```python
from build123d import *

# Parameters (mm, degrees)
EXTRUDE_1_DEPTH     = 20
SKETCH_2_W          = 23.1
SKETCH_2_H          = 23.1
SKETCH_2_W_2        = 15.1
SKETCH_2_H_2        = 15.1
EXTRUDE_2_DEPTH     = 24
SKETCH_3_W          = 4
SKETCH_3_H          = 23.1
EXTRUDE_3_DEPTH     = 15
SKETCH_4_R          = 1.8
CUT_EXTRUDE_1_DEPTH = 15
SKETCH_5_R          = 1.8
CUT_EXTRUDE_2_DEPTH = 35
SKETCH_6_W          = 23.1
SKETCH_6_H          = 19
CUT_EXTRUDE_3_DEPTH = 2


with BuildPart() as part:
    # 草图1 → 凸台-拉伸1 (new body)
    with BuildSketch(Plane(origin=(0, 0, 0), x_dir=(1, 0, 0), z_dir=(0, 1, 0))):
        Polygon((-11.153846154, 14.269230769), (-7.153846154, 14.269230769), (-7.153846154, -0.730769231), (7.946153846, -0.730769231), (7.946153846, 14.269230769), (11.946153846, 14.269230769), (11.946153846, -0.730769231), (11.946153846, -4.730769231), (-7.384615385, -4.730769231), (-11.153846154, -4.730769231), align=None)
    extrude(amount=EXTRUDE_1_DEPTH)

    # 草图2 → 凸台-拉伸2 (add)
    with BuildSketch(Plane(origin=(0, 0, 0.730769231), x_dir=(-1, 0, 0), z_dir=(0, 0, -1))):
        with Locations((-0.396153846, -11.55)):
            Rectangle(SKETCH_2_W, SKETCH_2_H)
        with Locations((-0.396153846, -11.55)):
            Rectangle(SKETCH_2_W_2, SKETCH_2_H_2, mode=Mode.SUBTRACT)
    extrude(amount=-EXTRUDE_2_DEPTH)

    # 草图3 → 凸台-拉伸3 (add)
    with BuildSketch(Plane(origin=(0, 0, 0.730769231), x_dir=(-1, 0, 0), z_dir=(0, 0, -1))):
        with Locations((-9.946153846, -11.55)):
            Rectangle(SKETCH_3_W, SKETCH_3_H)
        with Locations((9.153846154, -11.55)):
            Rectangle(SKETCH_3_W, SKETCH_3_H)
    extrude(amount=EXTRUDE_3_DEPTH)

    # 草图4 → 切除-拉伸1 (cut)
    with BuildSketch(Plane.XY.offset(4.730769231)):
        with Locations((0, 12.5)):
            Circle(SKETCH_4_R)
    extrude(amount=-CUT_EXTRUDE_1_DEPTH, mode=Mode.SUBTRACT)

    # 草图5 → 切除-拉伸2 (cut)
    with BuildSketch(Plane(origin=(11.946153846, 0, 0), x_dir=(0, 0, -1), z_dir=(1, 0, 0))):
        with Locations((-17.230769231, -11.5)):
            Circle(SKETCH_5_R)
    extrude(amount=-CUT_EXTRUDE_2_DEPTH, mode=Mode.SUBTRACT)

    # 草图6 → 切除-拉伸3 (cut)
    with BuildSketch(Plane(origin=(0, 20, 0), x_dir=(1, 0, 0), z_dir=(0, 1, 0))):
        with Locations((0.396153846, 4.769230769)):
            Rectangle(SKETCH_6_W, SKETCH_6_H)
    extrude(amount=-CUT_EXTRUDE_3_DEPTH, mode=Mode.SUBTRACT)


solid = part.part
```
For this review, take the finished solid that the model builds, in its own axes (mm). A direction names the side the tool comes from. Give positions to 0.01 mm unless a question says otherwise; leave off trailing zeros. Loops run counter-clockwise (first coordinate to the right, second up) from the corner with the lowest first, then second, coordinate; pieces in that order, holes last. Notation, with made-up numbers: M 19.25,-12 L 63.25,-12 A19 ccw 63.25,0 Z; hole C 10.5,89 d4. An arc over 180 degrees is marked long. One line per item, written item: value. Start each with the question number.
Q1. Add section D-D (y = 12.5). Give the boundary of the cut face in (x, z), and give its area (3 significant figures).
Q2. Add section B-B (x = 2.75). Give the boundary of the cut face in (y, z), and give its area (3 significant figures).
Q3. Add section A-A (y = -11.5). Give the boundary of the cut face in (x, z).
Q4. For L1, parallel to Y at x = 0, z = 3.75; L2, parallel to X at y = -16, z = 16.5; L3, parallel to Y at x = -5, z = 16, list the stretches that pass through material, from the lowest coordinate up.
Q5. Draft analysis for pull direction Y (two halves, no side actions). For faces 1 (the face through (-9.13, -11.42, 19.03)), 2 (the face through (1, 0, 15)), 3 (the face through (-7.154, -7, 1)), 4 (the face through (8.3, -11.4, 24.731)), state which applies: released by +Y, released by -Y, zero draft, split by the parting line, or undercut.
Q6. Add section C-C (z = 8). Give the boundary of the cut face in (x, y).
Q7. Clearance check with flat-ended pins moving along their axes: pin 1 Ø1.5 at (x, z) = (9, 8) entering from +Y; pin 2 Ø3 at (y, z) = (-11.5, 17.23) entering from -X; pin 3 Ø12 at (x, y) = (-0.5, 2.5) entering from -Z; pin 4 Ø5 at (x, z) = (-8, 6) entering from +Y. State where each tip first meets the part, or that it passes through.
Q8. Machinability: for faces 5 (the face through (1, 7, 0.731)), 6 (the face through (1, -4, 13)), 7 (the face through (0, 9, 4.731)), 8 (the face through (-2, 18, 1)), 9 (the face through (7.946, -7, 1)), which of the approach directions +Z, -Z, +X, -X, +Y, -Y give a long, thin tool a straight path to every point of the face, cutting with its end or side? Answer none if there is none.
Reply:
1. outline: M -11.15,-14.27 L -7.15,-14.27 L -7.15,0.73 L -1.8,0.73 L -1.8,4.73 L -11.15,4.73 Z; M 1.8,0.73 L 7.95,0.73 L 7.95,-14.27 L 11.95,-14.27 L 11.95,4.73 L 1.8,4.73 Z
1. area: 198 mm²
2. outline: M -23.1,0.73 L -19.1,0.73 L -19.1,24.73 L -23.1,24.73 Z; M -4,0.73 L 18,0.73 L 18,4.73 L 0,4.73 L 0,24.73 L -4,24.73 Z
2. area: 264 mm²
3. outline: M -11.15,-14.27 L -7.15,-14.27 L -7.15,15.43 L -11.15,15.43 Z; M -11.15,19.03 L -7.15,19.03 L -7.15,24.73 L -11.15,24.73 Z; M 7.95,-14.27 L 11.95,-14.27 L 11.95,15.43 L 7.95,15.43 Z; M 7.95,19.03 L 11.95,19.03 L 11.95,24.73 L 7.95,24.73 Z
4. L1: -23.1 to -19.1, -4 to 10.7, 14.3 to 18
4. L2: -11.15 to -7.15, 7.95 to 11.95
4. L3: -23.1 to -19.1, -4 to 0
5. face 1: undercut
5. face 2: released by +Y
5. face 3: undercut
5. face 4: zero draft
6. outline: M -11.15,-23.1 L 11.95,-23.1 L 11.95,0 L -11.15,0 Z; hole M -7.15,-19.1 L 7.95,-19.1 L 7.95,-4 L -7.15,-4 Z
7. pin 1: y = 0
7. pin 2: through
7. pin 3: z = 0.73
7. pin 4: y = 18
8. face 5: -Z, +Y, -Y
8. face 6: +Z, -Z
8. face 7: +Z, +X, -X, +Y
8. face 8: +Z, -Z, +X, -X, +Y
8. face 9: -Z
